```python
from build123d import *

# Parameters (mm, degrees)
SKETCH1_W           = 15
SKETCH1_H           = 10
BOSS_EXTRUDE2_DEPTH = 2
SKETCH2_R           = 2
CUT_EXTRUDE2_DEPTH  = 2
SKETCH3_W           = 2
SKETCH3_H           = 10
BOSS_EXTRUDE3_DEPTH = 33
SKETCH4_R           = 2
CUT_EXTRUDE3_DEPTH  = 33


with BuildPart() as part:
    # Sketch1 → Boss-Extrude2 (new body)
    with BuildSketch(Plane.XY):
        Rectangle(SKETCH1_W, SKETCH1_H)
    extrude(amount=BOSS_EXTRUDE2_DEPTH)

    # Sketch2 → Cut-Extrude2 (cut)
    with BuildSketch(Plane.XY.offset(2)):
        Circle(SKETCH2_R)
    extrude(amount=-CUT_EXTRUDE2_DEPTH, mode=Mode.SUBTRACT)

    # Sketch3 → Boss-Extrude3 (add)
    with BuildSketch(Plane.XY.offset(2)):
        with Locations((-6.5, 0)):
            Rectangle(SKETCH3_W, SKETCH3_H)
    extrude(amount=BOSS_EXTRUDE3_DEPTH)

    # Sketch4 → Cut-Extrude3 (cut)
    with BuildSketch(Plane(origin=(-5.5, 0, 0), x_dir=(0, 0, -1), z_dir=(1, 0, 0))):
        with Locations(Location((-25, 0, 0), (0, 0, 90))):
            Circle(SKETCH4_R)
    extrude(amount=-CUT_EXTRUDE3_DEPTH, mode=Mode.SUBTRACT)


solid = part.part
```
Can you work these out from the model? Positions are in its coordinate system, mm. A direction names the side the tool comes from. Coordinates: 2 decimals unless noted, no trailing zeros. Loops run counter-clockwise (first coordinate to the right, second up) from the corner with the lowest first, then second, coordinate; pieces in that order, holes last. Notation, with made-up numbers: (50, 14) -> (89, 14) arc R26 cw to (89, 46) -> close; hole circle Ø2 at (20.25, 41). An arc over 180 degrees is marked (long way). Answer as a JSON object with one key per item and string values.
1) Imagine slicing it at C-C (y = 0). Please give me the cut outline in (x, z).
Results:
{"outline": "(-7.5, 0) -> (-2, 0) -> (-2, 2) -> (-5.5, 2) -> (-5.5, 23) -> (-7.5, 23) -> close; (-7.5, 27) -> (-5.5, 27) -> (-5.5, 35) -> (-7.5, 35) -> close; (2, 0) -> (7.5, 0) -> (7.5, 2) -> (2, 2) -> close"}
2) Imagine slicing it at B-B (z = 25). Please give me the cut outline in (x, y), then the cut area to 3 significant figures.
Results:
{"outline": "(-7.5, -5) -> (-5.5, -5) -> (-5.5, -2) -> (-7.5, -2) -> close; (-7.5, 2) -> (-5.5, 2) -> (-5.5, 5) -> (-7.5, 5) -> close", "area": "12.0 mm^2"}
3) Thinking about a two-plate mould opening in Y: for faces 1 (the face through (2.4, 0.1, 2)), 2 (the face through (0, -2, 1)), 3 (the face through (-6, 0, 23)), 4 (the face through (-6, 5, 14)), which applies, pulls with the +Y half, pulls with the -Y half, needs draft (parallel to the pull), parting line crosses it, or undercut?
Results:
{"face 1": "needs draft", "face 2": "undercut", "face 3": "undercut", "face 4": "pulls with the +Y half"}
4) If I drill on line 1 (Z direction, x = -6.65, y = 0); line 2 (X direction, y = 4.5, z = 24.5); line 3 (Y direction, x = 0, z = 1.2), over which ranges is the centre line in solid material (lowest first)?
Results:
{"line 1": "z = 0 to 23, 27 to 35", "line 2": "x = -7.5 to -5.5", "line 3": "y = -5 to -2, 2 to 5"}
5) For P1, Ø3.5, axis at x = 0, y = 0, coming from the -Z side; P2, Ø3, axis at y = -3, z = 19, coming from the +X side, each with a flat end and sliding along its axis, tell me the tip position at first contact or that it passes through.
Results:
{"P1": "passes through", "P2": "stops at x = -5.5"}
6) Imagine slicing it at A-A (x = 0). Please give me the cut outline in (y, z).
Results:
{"outline": "(-5, 0) -> (-2, 0) -> (-2, 2) -> (-5, 2) -> close; (2, 0) -> (5, 0) -> (5, 2) -> (2, 2) -> close"}
7) For faces 5 (the face through (-7, 0, 35)), 6 (the face through (-5.5, 0, 18)), which set-ups out of +Z, -Z, +X, -X, +Y, -Y let a thin tool reach every point of the face, with its end or its side?
Results:
{"face 5": "+Z, +X, -X, +Y, -Y", "face 6": "+Z, +X, +Y, -Y"}
8) Imagine slicing it at D-D (x = -6.25). Please give me the cut outline in (y, z).
Results:
{"outline": "(-5, 0) -> (5, 0) -> (5, 35) -> (-5, 35) -> close; hole circle Ø4 at (0, 25)"}
